```python
from build123d import *

# Parameters (mm, degrees)
F2_R     = 5.5
F3_DEPTH = 25
F4_R     = 6.35
F5_DEPTH = 25


with BuildPart() as f1:
    # F0 (on Front) → F1 (revolve)
    with BuildSketch(Plane.XZ):
        Polygon((-38.1, 50), (-38.1, 40), (-35.1, 40), (-35.1, 10), (-38.1, 10), (-38.1, 0), (-35.1, 0), (-29.1, 0), (-29.1, 30), (0, 30), (0, 50), (-12.7, 50), (-18.1, 43), (-29.1, 43), (-36.1, 50), align=None)
    revolve(axis=Axis((0, 0, 40), (0, 0, -1)))

    # F2 (on face) → F3 (cut)
    with BuildSketch(Plane.XY.offset(43)):
        with Locations((-23.6, 0)):
            Circle(F2_R)
        with Locations((-16.68772, -16.68772)):
            Circle(F2_R)
        with Locations((0, -23.6)):
            Circle(F2_R)
        with Locations((16.68772, -16.68772)):
            Circle(F2_R)
        with Locations((23.6, 0)):
            Circle(F2_R)
        with Locations((16.68772, 16.68772)):
            Circle(F2_R)
        with Locations((0, 23.6)):
            Circle(F2_R)
        with Locations((-16.68772, 16.68772)):
            Circle(F2_R)
    extrude(amount=-F3_DEPTH, mode=Mode.SUBTRACT)

    # F4 (on face) → F5 (cut)
    with BuildSketch(Plane.XY.offset(50)):
        Circle(F4_R)
    extrude(amount=-F5_DEPTH, mode=Mode.SUBTRACT)


solid = f1.part
```
Model file for the job. Use its own axes, mm. A direction names the side the tool comes from. Coordinates: 2 decimals unless noted, no trailing zeros. Write each loop counter-clockwise with the first axis right and the second up, starting at its lowest first coordinate (ties: lowest second). Pieces come first, ordered by that corner, then holes. Notation, with made-up numbers: (-34, -6.75) - (9, -6.75) arc R11 ccw to (9, 3.25) - close; hole circle Ø9 at (60.25, -6.5). An arc over 180 degrees is marked (long way). Use a Markdown table: item, result. Add a question column.
Item 1: Band-saw the part on B-B, the plane y = 4. Give the number of separate pieces and of enclosed holes in the cut face, and give its area (3 significant figures).
Item 2: Two-plate mould, pull along X, no slides. Class faces 1 (the face through (30.235, -23.183, 44.93)), 2 (the face through (17, -31, 10)), 3 (the face through (-10, -22, 43)): pulls with the +X half, pulls with the -X half, needs draft (parallel to the pull), parting line crosses it, or undercut.
Item 3: 3-axis set-ups, long thin cutter, end or side, ignore diameter. For faces 4 (the face through (-10, 22, 43)), 5 (the face through (-6, -6, 30)), 6 (the face through (9, -28, 0)): which of +Z, -Z, +X, -X, +Y, -Y reach the whole face in a straight line?
Item 4: Band-saw the part on A-A, the plane z = 27.5. Write the cut outline in (x, y).
Item 5: Drill centre lines: line 1 along X through (y, z) = (0.5, 31.5); line 2 along Z through (x, y) = (25.5, 9); line 3 along Y through (x, z) = (4.5, 17). Where is each one in solid material? Low to high.
Item 6: Drop flat-ended pins along their axis: pin 1 (16.5 mm diameter, centred on x = 0, y = 0, fed in from -Z); pin 2 (13 mm diameter, centred on x = 25, y = -8.5, fed in from +Z); pin 3 (6 mm diameter, centred on y = 7, z = 8.5, fed in from -X). Give the stop position or say it passes through.
A:
| question | item | result |
|---|---|---|
| 1 | separate pieces | 4 |
| 1 | enclosed holes | 0 |
| 1 | area | 1,240 mm² |
| 2 | face 1 | parting line crosses it |
| 2 | face 2 | needs draft |
| 2 | face 3 | undercut |
| 3 | face 4 | +Z |
| 3 | face 5 | -Z |
| 3 | face 6 | -Z, +X, -X, +Y, -Y |
| 4 | outline | circle Ø70.2 at (0, 0); hole circle Ø58.2 at (0, 0) |
| 5 | line 1 | x = -35.1 to -29.08, -18.12 to -6.33, 6.33 to 18.12, 29.08 to 35.1 |
| 5 | line 2 | z = 30 to 43 |
| 5 | line 3 | y = -34.81 to -28.75, 28.75 to 34.81 |
| 6 | pin 1 | stops at z = 30 |
| 6 | pin 2 | stops at z = 46.81 |
| 6 | pin 3 | stops at x = -37.89 |
